```python
from build123d import *

# Parameters (mm, degrees)
SKETCH_1_R          = 9.5
SKETCH_1_R_2        = 0.85
EXTRUDE_1_DEPTH     = 1.4
SKETCH_2_R          = 3.85
SKETCH_2_R_2        = 3.1
CUT_EXTRUDE_1_DEPTH = 0.7
EXTRUDE_2_DEPTH     = 3


with BuildPart() as part:
    # 스케치1 → 보스-돌출1 (new body)
    with BuildSketch(Plane(origin=(0, 0, 0), x_dir=(1, 0, 0), z_dir=(0, 1, 0))):
        with Locations(Location((0, 0, 0), (0, 0, 270))):
            Circle(SKETCH_1_R)
        with Locations(Location((0, 7, 0), (0, 0, 270))):
            Circle(SKETCH_1_R_2, mode=Mode.SUBTRACT)
        with Locations(Location((3.5, 6.062177826, 0), (0, 0, 270))):
            Circle(SKETCH_1_R_2, mode=Mode.SUBTRACT)
        with Locations(Location((6.062177826, 3.5, 0), (0, 0, 270))):
            Circle(SKETCH_1_R_2, mode=Mode.SUBTRACT)
        with Locations(Location((7, 0, 0), (0, 0, 270))):
            Circle(SKETCH_1_R_2, mode=Mode.SUBTRACT)
        with Locations(Location((6.062177826, -3.5, 0), (0, 0, 270))):
            Circle(SKETCH_1_R_2, mode=Mode.SUBTRACT)
        with Locations(Location((3.5, -6.062177826, 0), (0, 0, 270))):
            Circle(SKETCH_1_R_2, mode=Mode.SUBTRACT)
        with Locations(Location((0, -7, 0), (0, 0, 270))):
            Circle(SKETCH_1_R_2, mode=Mode.SUBTRACT)
        with Locations(Location((-3.5, -6.062177826, 0), (0, 0, 270))):
            Circle(SKETCH_1_R_2, mode=Mode.SUBTRACT)
        with Locations(Location((-6.062177826, -3.5, 0), (0, 0, 270))):
            Circle(SKETCH_1_R_2, mode=Mode.SUBTRACT)
        with Locations(Location((-7, 0, 0), (0, 0, 270))):
            Circle(SKETCH_1_R_2, mode=Mode.SUBTRACT)
        with Locations(Location((-6.062177826, 3.5, 0), (0, 0, 270))):
            Circle(SKETCH_1_R_2, mode=Mode.SUBTRACT)
        with Locations(Location((-3.5, 6.062177826, 0), (0, 0, 270))):
            Circle(SKETCH_1_R_2, mode=Mode.SUBTRACT)
    extrude(amount=EXTRUDE_1_DEPTH)

    # 스케치2 → 컷-돌출1 (cut)
    with BuildSketch(Plane(origin=(0, 1.4, 0), x_dir=(1, 0, 0), z_dir=(0, 1, 0))):
        with Locations(Location((0, 0, 0), (0, 0, 270))):
            Circle(SKETCH_2_R)
        with Locations(Location((0, 0, 0), (0, 0, 270))):
            Circle(SKETCH_2_R_2, mode=Mode.SUBTRACT)
    extrude(amount=-CUT_EXTRUDE_1_DEPTH, mode=Mode.SUBTRACT)

    # 스케치3 → 보스-돌출2 (add)
    with BuildSketch(Plane.XZ):
        with BuildLine():
            Line((-0.8, 2.891366459), (-0.8, 3.8))
            Line((-0.8, 3.8), (0.8, 3.8))
            Line((0.8, 3.8), (0.8, 2.891366459))
            ThreePointArc((0.8, 2.891366459), (0, -3), (-0.8, 2.891366459))
        make_face()
    extrude(amount=EXTRUDE_2_DEPTH)


solid = part.part
```
For this review, take the finished solid that the model builds, in its own axes (mm). A direction names the side the tool comes from. Round coordinates to 2 decimals unless told otherwise and drop trailing zeros. Loops run counter-clockwise (first coordinate to the right, second up) from the corner with the lowest first, then second, coordinate; pieces in that order, holes last.
Q1. Mouldability with a two-part tool opening along X and no side actions: class faces 4 (the face through (2, 0.7, -3)), 5 (the face through (0.8, -1.5, 3.4)), 6 (the face through (0.1, 1.4, 4.1)) as +X half, -X half, draft (parallel to the pull), parting line (faces both ways), or undercut.
Result sheet:
face 4: undercut
face 5: +X half
face 6: draft
Q2. To check wall thickness, follow line 1 along X through (y, z) = (1.1, 0); line 2 along Z through (x, y) = (1.25, 1); line 3 along Z through (x, y) = (-6.25, 0.6). State the ranges of each line that lie inside material, in increasing order.
Result sheet:
line 1: x = -9.5 to -7.85, -6.15 to -3.85, -3.1 to 3.1, 3.85 to 6.15, 7.85 to 9.5
line 2: z = -9.42 to -3.64, -2.84 to 2.84, 3.64 to 9.42
line 3: z = -7.15 to -4.33, -2.67 to -0.4, 0.4 to 2.67, 4.33 to 7.15
Q3. Machinability: for faces 1 (the face through (0, -1, 3.8)), 2 (the face through (-0.8, -1.5, 3.3)), 3 (the face through (0, -1, -3)), which of the approach directions +Z, -Z, +X, -X, +Y, -Y give a long, thin tool a straight path to every point of the face, cutting with its end or side? Answer none if there is none.
Result sheet:
face 1: +Z, +X, -X, -Y
face 2: +Z, -X, -Y
face 3: -Y
Q4. Insertion check: pin 1 Ø2 at (x, z) = (7, 0) entering from -Y; pin 2 Ø2 at (y, z) = (-1.5, -0.5) entering from +X; pin 3 Ø0.8 at (x, y) = (0, -1) entering from +Z. Each pin has a flat end and moves straight along its axis. Give the tip position at first contact, or say it passes through.
Result sheet:
pin 1: stops at y = 0
pin 2: stops at x = 3
pin 3: stops at z = 3.8
Q5. Add section C-C on z = -7.5. Write out the cut boundary in (x, y).
Result sheet:
outline: (-5.83, 0) - (-0.69, 0) - (-0.69, 1.4) - (-5.83, 1.4) - close; (0.69, 0) - (5.83, 0) - (5.83, 1.4) - (0.69, 1.4) - close
Q6. Add section A-A on x = 0. Write out the cut boundary in (y, z), plus the area to 3 significant figures.
Result sheet:
outline: (-3, -3) - (0, -3) - (0, -6.15) - (1.4, -6.15) - (1.4, -3.85) - (0.7, -3.85) - (0.7, -3.1) - (1.4, -3.1) - (1.4, 3.1) - (0.7, 3.1) - (0.7, 3.85) - (1.4, 3.85) - (1.4, 6.15) - (0, 6.15) - (0, 3.8) - (-3, 3.8) - close; (0, -9.5) - (1.4, -9.5) - (1.4, -7.85) - (0, -7.85) - close; (0, 7.85) - (1.4, 7.85) - (1.4, 9.5) - (0, 9.5) - close
area: 41.2 mm2
Q7. Add section B-B on z = 0. Write out the cut boundary in (x, y).
Result sheet:
outline: (-9.5, 0) - (-7.85, 0) - (-7.85, 1.4) - (-9.5, 1.4) - close; (-6.15, 0) - (-3, 0) - (-3, -3) - (3, -3) - (3, 0) - (6.15, 0) - (6.15, 1.4) - (3.85, 1.4) - (3.85, 0.7) - (3.1, 0.7) - (3.1, 1.4) - (-3.1, 1.4) - (-3.1, 0.7) - (-3.85, 0.7) - (-3.85, 1.4) - (-6.15, 1.4) - close; (7.85, 0) - (9.5, 0) - (9.5, 1.4) - (7.85, 1.4) - close
Q8. Add section D-D on y = -1.15. Write out the cut boundary in (x, z).
Result sheet:
outline: (-0.8, 2.89) arc R3 ccw (long way) to (0.8, 2.89) - (0.8, 3.8) - (-0.8, 3.8) - close
